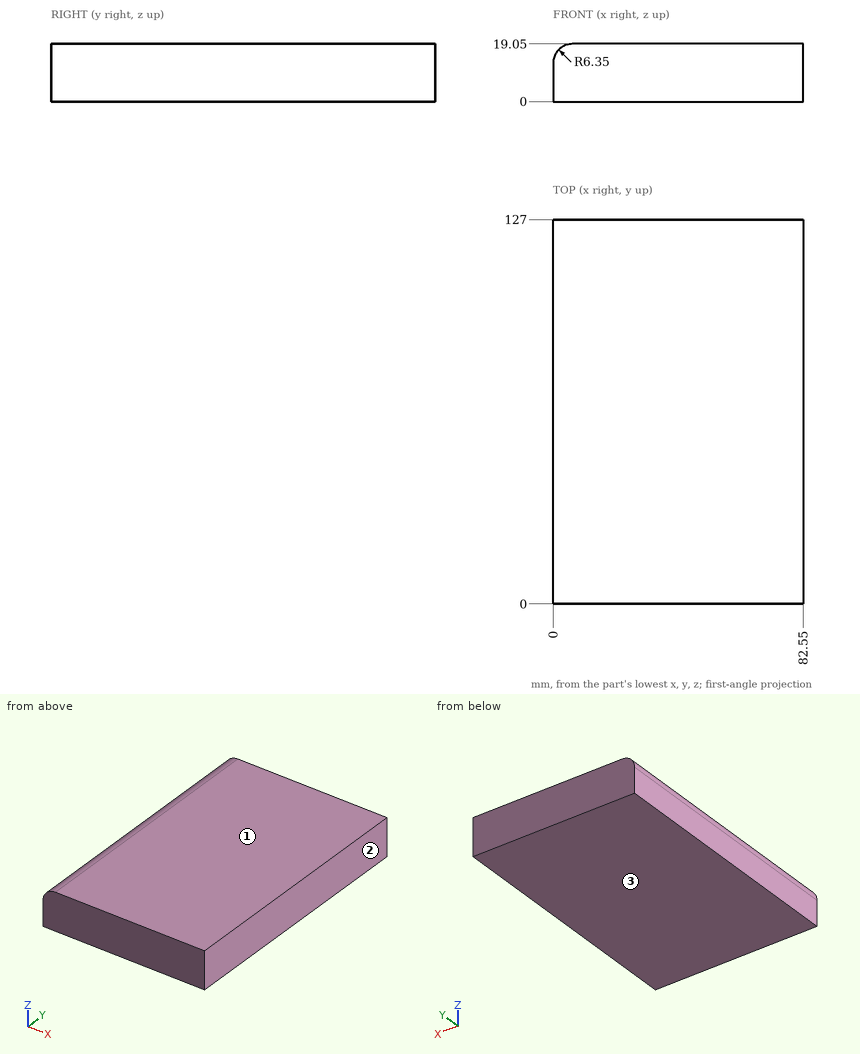
Check sheet for the drawn part. Datum: minimum x, y, z corner. Units: mm. Round coordinates to 2 decimals unless told otherwise and drop trailing zeros. Write each question's results on one line, items separated by ' | '.
1) Gauge pin test, flat end, axial feed: P1, Ø3, axis at y = 58.5, z = 15.5, coming from the -X side. Record the tip position at first contact, or that the pin passes through.
Checks:
P1: stops at x = 0.13
2) Mould release check, pull along Z, two halves, no side actions. Record for the marked faces 1, 2 and 3: released by +Z, released by -Z, zero draft, split by the parting line, or undercut.
Checks:
face 1: released by +Z | face 2: zero draft | face 3: released by -Z
3) Scan lines: L1, parallel to X at y = 112, z = 15.5; L2, parallel to X at y = 26.5, z = 16.25. Record each from-to range of solid material in increasing order. Write a range as from..to.
Checks:
L1: x = 0.65..82.55 | L2: x = 1.09..82.55
